```python
from build123d import *

# Parameters (mm, degrees)
RESSALTO_EXTRUS_O1_DEPTH = 12
ESBO_O4_W                = 8
ESBO_O4_H                = 20.4
RESSALTO_EXTRUS_O2_DEPTH = 3
CASCA2_T                 = -0.8
ESBO_O5_R                = 1.65
RESSALTO_EXTRUS_O3_DEPTH = 2.5


with BuildPart() as part:
    # Esboço1 → Ressalto-extrusão1 (new body, symmetric)
    with BuildSketch(Plane.XY):
        with BuildLine():
            Line((-5, 0), (5, 0))
            Line((5, 0), (5, -1.5))
            ThreePointArc((5, -1.5), (5.050220269, -2.256637298), (5.2, -3))
            Line((5.2, -3), (2.890598923, -7))
            Line((2.890598923, -7), (1, -7))
            ThreePointArc((1, -7), (-3.242640687, -5.242640687), (-5, -1))
            Line((-5, -1), (-5, 0))
        make_face()
    extrude(amount=RESSALTO_EXTRUS_O1_DEPTH, both=True)

    # Esboço4 → Ressalto-extrusão2 (add)
    with BuildSketch(Plane(origin=(0, 0, 0), x_dir=(1, 0, 0), z_dir=(0, 1, 0))):
        with Locations((0, -0.2)):
            Rectangle(ESBO_O4_W, ESBO_O4_H)
    extrude(amount=RESSALTO_EXTRUS_O2_DEPTH)

    # Casca2
    casca2_openings = [part.faces().sort_by_distance(p)[0] for p in [
        (4.045299462, -5, 0),
        (0, 3, 0.2),
    ]]
    offset(amount=CASCA2_T, openings=casca2_openings, kind=Kind.INTERSECTION)

    # Esboço5 → Ressalto-extrusão3 (add)
    with BuildSketch(Plane(origin=(0, 0, 0), x_dir=(0, 0, -1), z_dir=(1, 0, 0))):
        with BuildLine():
            Line((-12, 0), (-12.5, 0))
            Line((-12.5, 0), (-12.5, 3))
            ThreePointArc((-12.5, 3), (-13.232233047, 4.767766953), (-15, 5.5))
            Line((-15, 5.5), (-18, 5.5))
            Line((-18, 5.5), (-18, -5))
            Line((-18, -5), (-12, -5))
            Line((-12, -5), (-12, 0))
        make_face()
        with Locations((-15, 3)):
            Circle(ESBO_O5_R, mode=Mode.SUBTRACT)
    extrude(amount=RESSALTO_EXTRUS_O3_DEPTH)


solid = part.part
```
Could you check a few things on this model? Use its own coordinates, in mm. A direction names the side the tool comes from. Round coordinates to 2 decimals unless told otherwise and drop trailing zeros. Write each loop counter-clockwise with the first axis right and the second up, starting at its lowest first coordinate (ties: lowest second). Pieces come first, ordered by that corner, then holes.
(1) Suppose I cut it at C-C on x = -2.5. Write out the boundary of the cut face in (y, z), and give its area (3 significant figures).
Findings below:
outline: (-5.87, -12) - (0, -12) - (0, -10) - (3, -10) - (3, -9.2) - (-0.8, -9.2) - (-0.8, -11.2) - (-4.85, -11.2) - (-4.85, 11.2) - (-0.8, 11.2) - (-0.8, 9.6) - (3, 9.6) - (3, 10.4) - (0, 10.4) - (0, 12) - (-5.87, 12) - close
area: 40.1 mm2
(2) Suppose I cut it at A-A on z = 9.25. Write out the boundary of the cut face in (x, y) (3 decimals).
Findings below:
outline: (-5, -1) arc R6 ccw to (1, -7) - (2.891, -7) - (3.352, -6.2) - (1, -6.2) arc R5.2 cw to (-4.2, -1) - (-4.2, -0.8) - (-3.2, -0.8) - (-3.2, 3) - (-4, 3) - (-4, 0) - (-5, 0) - close; (3.2, -0.8) - (4.2, -0.8) - (4.2, -1.5) arc R6.525 ccw to (4.667, -3.924) - (5.2, -3) arc R5.725 cw to (5, -1.5) - (5, 0) - (4, 0) - (4, 3) - (3.2, 3) - close
(3) Thinking about a two-plate mould opening in Y: for faces 4 (the face through (0, -3, -11.2)), 5 (the face through (0, -3, -12)), 6 (the face through (-3.196, -5.289, 0.168)), which applies, +Y half, -Y half, draft (parallel to the pull), parting line (faces both ways), or undercut?
Findings below:
face 4: undercut
face 5: draft
face 6: -Y half
(4) Suppose I cut it at B-B on x = 2. Write out the boundary of the cut face in (y, z), and give its area (3 significant figures).
Findings below:
outline: (-7, -12) - (0, -12) - (0, -10) - (3, -10) - (3, -9.2) - (-0.8, -9.2) - (-0.8, -11.2) - (-6.2, -11.2) - (-6.2, 11.2) - (-0.8, 11.2) - (-0.8, 9.6) - (3, 9.6) - (3, 10.4) - (0, 10.4) - (0, 12.5) - (3, 12.5) arc R2.5 ccw to (5.5, 15) - (5.5, 18) - (-5, 18) - (-5, 12) - (-7, 12) - close; hole circle Ø3.3 at (3, 15)
area: 87.2 mm2
(5) Which directions (+Z, -Z, +X, -X, +Y, -Y) give clear straight access to the entire face, cutting with the end or side of a thin tool? Please do faces 1 (the face through (3.2, 1, 0)), 2 (the face through (0, -3, 11.2)), 3 (the face through (1, -5, 15)).
Findings below:
face 1: +Y
face 2: none
face 3: +Z, +X, -X, -Y
(6) If I drill on probe 1 along Y at (x, z) = (0.6, 15); probe 2 along Z at (x, y) = (-2.5, -2.25); probe 3 along X at (y, z) = (-0.75, -9), over which ranges is the centre line in solid material (lowest first)?
Findings below:
probe 1: y = -5 to 1.35, 4.65 to 5.5
probe 2: z = -12 to -11.2, 11.2 to 12
probe 3: x = -5 to -3.2, 3.2 to 5
(7) For pin 1 (1.5 mm diameter, centred on x = 0.5, y = 1.5, fed in from -Z); pin 2 (2.5 mm diameter, centred on x = 2.5, z = 0, fed in from +Y); pin 3 (1.5 mm diameter, centred on x = -3, y = 1, fed in from +Z); pin 4 (2 mm diameter, centred on y = 3, z = 15, fed in from +X), each with a flat end and sliding along its axis, tell me the tip position at first contact or that it passes through.
Findings below:
pin 1: stops at z = -10
pin 2: stops at y = 3
pin 3: stops at z = 10.4
pin 4: passes through
